Geometry: see drawing. Coordinates: mm, zero at the bounding-box minimum. Round coordinates to 2 decimals unless told otherwise and drop trailing zeros. Write each loop counter-clockwise with the first axis right and the second up, starting at its lowest first coordinate (ties: lowest second). Pieces come first, ordered by that corner, then holes. Notation, with made-up numbers: M 69.5,32 L 111.5,32 A29 cw 111.5,60 Z; hole C 76.5,55 d3. An arc over 180 degrees is marked long. Use one line per item in the form item = value. Start each with the question number.
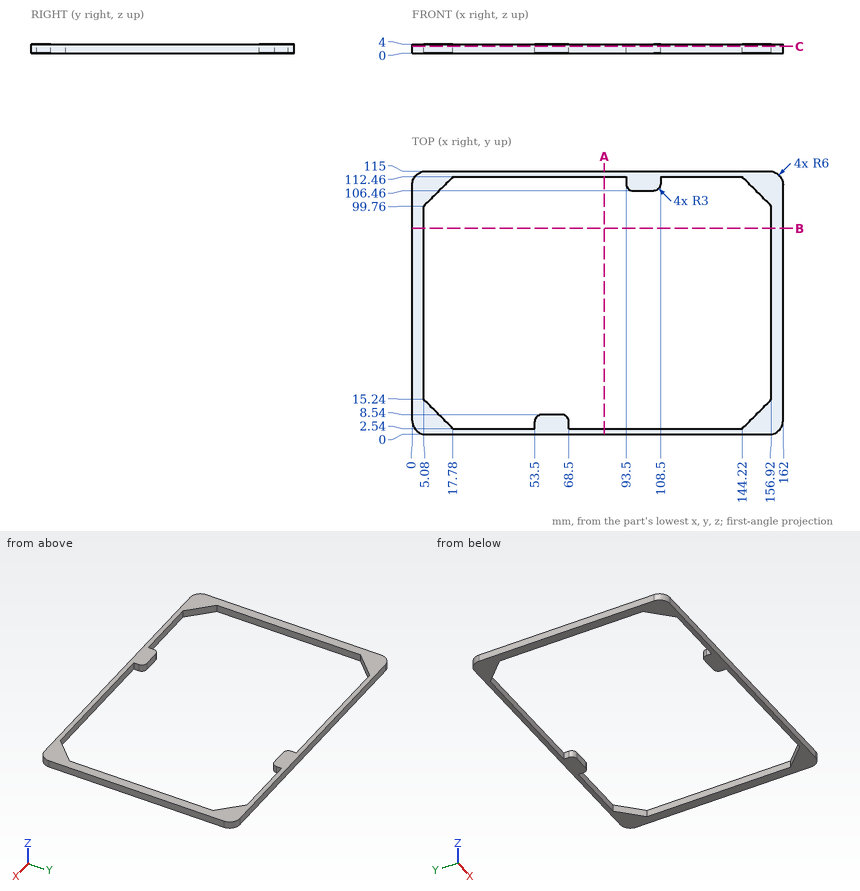
Item 1: Cut plane C-C (z = 2.95). Output: boundary loops of the cut face in (x, y), plus the area to 3 significant figures.
Item 2: First-contact query: pin 1 (1 mm diameter, centred on x = 84.5, z = 2, fed in from -Y); pin 2 (0.9 mm diameter, centred on y = 3.5, z = 3, fed in from +X); pin 3 (0.9 mm diameter, centred on y = 110.5, z = 1, fed in from -X). Flat tips, straight axial feed; report the tip coordinate or a pass-through.
Item 3: Cut plane A-A (x = 84). Output: boundary loops of the cut face in (y, z), plus the area to 3 significant figures.
Item 4: Cut plane B-B (y = 90). Output: boundary loops of the cut face in (x, z), plus the area to 3 significant figures.
Item 5: Ray query, line 1 (Y direction, x = 99, z = 1.6); line 2 (X direction, y = 43.5, z = 2.1); line 3 (Y direction, x = 127, z = 3.1). Return the intervals inside material, ascending. Write a range as from..to.
Final values:
q1.outline = M 0,6 A6 ccw 6,0 L 156,0 A6 ccw 162,6 L 162,109 A6 ccw 156,115 L 6,115 A6 ccw 0,109 Z; hole M 5.08,15.24 L 17.78,2.54 L 53.5,2.54 L 53.5,5.54 A3 cw 56.5,8.54 L 65.5,8.54 A3 cw 68.5,5.54 L 68.5,2.54 L 144.22,2.54 L 156.92,15.24 L 156.92,99.76 L 144.22,112.46 L 108.5,112.46 L 108.5,109.46 A3 cw 105.5,106.46 L 96.5,106.46 A3 cw 93.5,109.46 L 93.5,112.46 L 17.78,112.46 L 5.08,99.76 Z
q1.area = 2,400 mm^2
q2.pin_1 = 0
q2.pin_2 = 161.64
q2.pin_3 = 0.09
q3.outline = M 0,0 L 2.54,0 L 2.54,4 L 0,4 Z; M 112.46,0 L 115,0 L 115,4 L 112.46,4 Z
q3.area = 20.3 mm^2
q4.outline = M 0,0 L 5.08,0 L 5.08,4 L 0,4 Z; M 156.92,0 L 162,0 L 162,4 L 156.92,4 Z
q4.area = 40.6 mm^2
q5.line_1 = 0..2.54, 106.46..115
q5.line_2 = 0..5.08, 156.92..162
q5.line_3 = 0..2.54, 112.46..115
